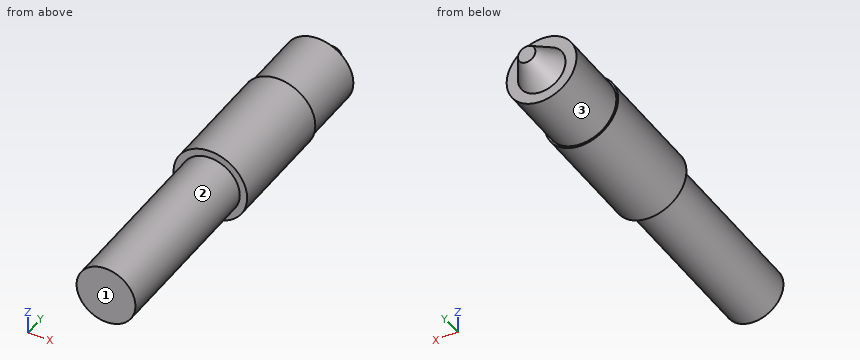
```python
from build123d import *

# Parameters (mm, degrees)
F0_R     = 10
F1_DEPTH = 105
F2_R     = 15.829985
F2_R_2   = 9.5
F3_DEPTH = 25.3
F6_R     = 17.927182
F6_R_2   = 8
F7_DEPTH = 48.2


with BuildPart() as f1:
    # F0 (on Front) → F1 (new body)
    with BuildSketch(Plane.XZ):
        Circle(F0_R)
    extrude(amount=F1_DEPTH)

    # F2 (on face) → F3 (cut)
    with BuildSketch(Plane(origin=(0, 0, 0), x_dir=(-1, 0, 0), z_dir=(0, 1, 0))):
        Circle(F2_R)
        Circle(F2_R_2, mode=Mode.SUBTRACT)
    extrude(amount=-F3_DEPTH, mode=Mode.SUBTRACT)

    # F4 (on Right) → F5 (revolve, cut)
    with BuildSketch(Plane.YZ):
        Polygon((-7, 17.069709), (-7, 6.35), (3.998523, 0), (6.907294, 0.035041), (6.702085, 17.069709), align=None)
    revolve(axis=Axis((0, 5.452908, 0.01752), (0, 0.999927, 0.012046)), mode=Mode.SUBTRACT)

    # F6 (on face) → F7 (cut)
    with BuildSketch(Plane.XZ.offset(105)):
        Circle(F6_R)
        Circle(F6_R_2, mode=Mode.SUBTRACT)
    extrude(amount=-F7_DEPTH, mode=Mode.SUBTRACT)


solid = f1.part
```
Input: part model. Units: mm. Frame: model coordinates. Face numbers are marked on the shaded views. A direction names the side the tool comes from. Coordinates: 2 decimals unless noted, no trailing zeros. Write each loop counter-clockwise with the first axis right and the second up, starting at its lowest first coordinate (ties: lowest second). Pieces come first, ordered by that corner, then holes.
1) Set-up query: the marked faces 1, 2 and 3. Return all of +Z, -Z, +X, -X, +Y, -Y with unobstructed straight access to the full face (end or side cutting, diameter ignored); none if empty.
2) Section C-C on y = -87. Output: boundary loops of the cut face in (x, z).
3) Section B-B on y = -19. Output: boundary loops of the cut face in (x, z), and give its area (3 significant figures).
4) Material intervals for line 1 along X through (y, z) = (-84.5, 0.5); line 2 along Z through (x, y) = (-0.5, -13), sorted ascending.
5) Pin query (flat end, axial travel): pin 1 Ø1.5 at (x, z) = (-7, -0.5) entering from +Y; pin 2 Ø10 at (x, z) = (-3.5, 4.5) entering from +Y; pin 3 Ø8 at (y, z) = (-15.5, -6) entering from -X; pin 4 Ø2 at (x, y) = (-3.5, -78) entering from +Z. Return the tip coordinate at first contact, or that it passes through.
6) Section A-A on x = 0. Output: boundary loops of the cut face in (y, z).
Check result:
1. face 1: +Z, -Z, +X, -X, -Y
1. face 2: -Y
1. face 3: +Y
2. outline: circle Ø16 at (0, 0)
3. outline: circle Ø19 at (0, 0)
3. area: 284 mm2
4. line 1: x = -7.98 to 7.98
4. line 2: z = -9.49 to 9.49
5. pin 1: stops at y = -6.54
5. pin 2: stops at y = 0
5. pin 3: stops at x = -9.29
5. pin 4: stops at z = 7.6
6. outline: (-105, -8) - (-56.8, -8) - (-56.8, -10) - (-25.3, -10) - (-25.3, -9.5) - (-6.77, -9.5) - (-6.84, -6.61) - (0, -2.44) - (0, 2.31) - (-7, 6.35) - (-7, 9.5) - (-25.3, 9.5) - (-25.3, 10) - (-56.8, 10) - (-56.8, 8) - (-105, 8) - close
